Autodesk Fusion 360 part; units mm, degrees
sketch "Sketch2" plane through (0, 0, 0) normal (0, 1, 0) x (1, 0, 0)
  line L0 (0, 0) -> (-28, 0)
  line L1 (-28, 0) -> (-28, 28)
  line L2 (-28, 28) -> (0, 28)
  line L3 (0, 28) -> (0, 0)
  dimension "d1" = 28
  dimension "d2" = 28
extrude "Extrude1" add sketch "Sketch2" along normal blind 635
sketch "Sketch3" plane through (0, 0, -28) normal (0, 0, -1) x (-1, 0, 0)
  line L0 (0, 0) -> (28, 0)
  line L1 (28, 0) -> (28, 635)
  line L2 (28, 635) -> (0, 635)
  line L3 (0, 635) -> (0, 0)
  circle A0 centre (13, 620) radius 6
  line L4 (28, 317.5) -> (0, 317.5) construction
  circle A1 centre (13, 15) radius 6
  dimension "d5" = 12
  dimension "d6" = 15
  dimension "d7" = 15
extrude "Extrude2" cut sketch "Sketch3" against normal through all contours A0 | A1
fillet "Fillet1" radius 0.5 12 edges at (-28, 317.5, 0) (0, 317.5, 0) (-28, 317.5, -28) (0, 317.5, -28) (0, 635, -14) (-14, 635, -28) (-28, 635, -14) (-14, 635, 0) (-14, 0, 0) (-28, 0, -14) (0, 0, -14) (-14, 0, -28)
equation "d7 = d6"
Build history of the part. All positions in model axes, mm. Round coordinates to 2 decimals unless told otherwise and drop trailing zeros. Order: outer loops, then holes, each group sorted by start corner. A loop starts at its lowest first (then second) coordinate and runs counter-clockwise, first axis right, second up. Notation, with made-up numbers: M 7,16.25 L 11,16.25 A8 ccw 11,31.25 Z; hole C 8.5,-10 d11. An arc over 180 degrees is marked long. Use CSV: the item, a comma, the result in double quotes. Start each with the question number.
(1) Cut at A-A on y = 620. List the corners of the cut face in (x, z), then the cut area to 3 significant figures.
(2) Drill centre lines: probe 1 along Y at (x, z) = (-13, -16.25); probe 2 along Y at (x, z) = (-17.75, -20.5). Where is each one in solid material? Low to high.
(3) Cut at B-B on x = -13. List the corners of the cut face in (y, z), then the cut area to 3 significant figures.
(4) Flat gauge pin, fed straight in: P1, Ø2, axis at x = -13.5, y = 412, coming from the +Z side. Where does the tip first touch, or does it go through?
(5) Mould opens along X. For faces 1 (the face through (-14, 313, -28)), 2 (the face through (-12.22, 625.95, -14.2)), 3 (the face through (-28, 313, -14)) say: +X half, -X half, draft (parallel to the pull), parting line (faces both ways), or undercut.
Findings:
1,outline,"M -28,-27.5 A0.5 ccw -27.5,-28 L -19,-28 L -19,0 L -27.5,0 A0.5 ccw -28,-0.5 Z; M -7,-28 L -0.5,-28 A0.5 ccw 0,-27.5 L 0,-0.5 A0.5 ccw -0.5,0 L -7,0 Z"
1,area,"448 mm^2"
2,probe 1,"y = 0 to 9, 21 to 614, 626 to 635"
2,probe 2,"y = 0 to 11.33, 18.67 to 616.33, 623.67 to 635"
3,outline,"M 0,-27.5 A0.5 ccw 0.5,-28 L 9,-28 L 9,0 L 0.5,0 A0.5 ccw 0,-0.5 Z; M 21,-28 L 614,-28 L 614,0 L 21,0 Z; M 626,-28 L 634.5,-28 A0.5 ccw 635,-27.5 L 635,-0.5 A0.5 ccw 634.5,0 L 626,0 Z"
3,area,"17,100 mm^2"
4,P1,"stops at z = 0"
5,face 1,"draft"
5,face 2,"undercut"
5,face 3,"-X half"
